Geometry check sheet. Reference: drawing and pictorial views, mm from the part's lowest x, y, z. A direction names the side the tool comes from. Round coordinates to 2 decimals unless told otherwise and drop trailing zeros. Order: outer loops, then holes, each group sorted by start corner. A loop starts at its lowest first (then second) coordinate and runs counter-clockwise, first axis right, second up.
(1) Go/stop test with flat-tipped pins: pin 1 (1 mm diameter, centred on y = 65, z = 505, fed in from +X); pin 2 (1.5 mm diameter, centred on y = 132, z = 157.5, fed in from -X). Record where each tip stops, or that it passes through.
(2) Sectioned sample at B-B (x = 174). Record the boundary of the cut face in (y, z).
(3) Release check for a two-part mould opening along Z. For the marked faces 1, 2 and 3 record: +Z half, -Z half, draft (parallel to the pull), parting line (faces both ways), or undercut.
(4) Sectioned sample at C-C (z = 736.5). Record the boundary of the cut face in (x, y).
(5) Set-up check for the marked faces 4, 5 and 6: record each of +Z, -Z, +X, -X, +Y, -Y from which the full face is reachable in a straight line by a thin tool's end or side.
(6) Material ranges on line 1 along Z through (x, y) = (126.5, 174); line 2 along X through (y, z) = (73, 862); line 3 along Y through (x, z) = (517, 775.5), recorded low to high.
(7) Sectioned sample at A-A (y = 95). Record the boundary of the cut face in (x, z).
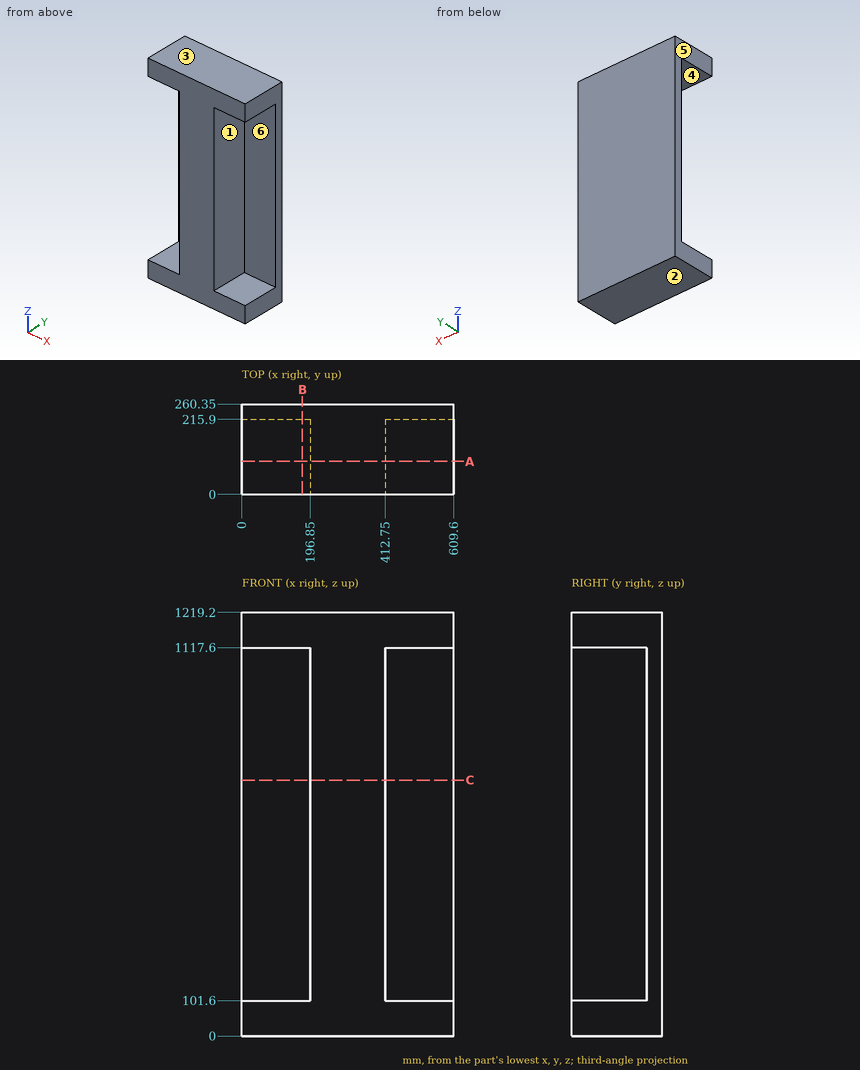
Answer below:
1. pin 1: stops at x = 412.75
1. pin 2: stops at x = 196.85
2. outline: (0, 0) - (260.35, 0) - (260.35, 1219.2) - (0, 1219.2) - (0, 1117.6) - (215.9, 1117.6) - (215.9, 101.6) - (0, 101.6) - close
3. face 1: undercut
3. face 2: -Z half
3. face 3: +Z half
4. outline: (0, 215.9) - (196.85, 215.9) - (196.85, 0) - (412.75, 0) - (412.75, 215.9) - (609.6, 215.9) - (609.6, 260.35) - (0, 260.35) - close
5. face 4: -X, -Y
5. face 5: +Z, -Z, -X, +Y, -Y
5. face 6: +X, -Y
6. line 1: z = 0 to 101.6, 1117.6 to 1219.2
6. line 2: x = 196.85 to 412.75
6. line 3: y = 215.9 to 260.35
7. outline: (0, 0) - (609.6, 0) - (609.6, 101.6) - (412.75, 101.6) - (412.75, 1117.6) - (609.6, 1117.6) - (609.6, 1219.2) - (0, 1219.2) - (0, 1117.6) - (196.85, 1117.6) - (196.85, 101.6) - (0, 101.6) - close
